Build history of the part. All positions in model axes, mm. Face numbers are marked on the shaded views. Round coordinates to 2 decimals unless told otherwise and drop trailing zeros. Order: outer loops, then holes, each group sorted by start corner. A loop starts at its lowest first (then second) coordinate and runs counter-clockwise, first axis right, second up. Notation, with made-up numbers: (77.5, 42.25) -> (81.5, 42.25) arc R10 cw to (81.5, 61.25) -> close; hole circle Ø8 at (69, 42.5). An arc over 180 degrees is marked (long way). Use a Markdown table: item, result. Add a question column.
Item 1: Two-plate mould, pull along Z, no slides. Class the marked faces 1, 2 and 3: released by +Z, released by -Z, zero draft, split by the parting line, or undercut.
Item 2: Slice it at A-A, the plane y = 0. Give the cut face in (x, z), plus the area to 3 significant figures.
Item 3: Slice it at D-D, the plane y = -13.5. Give the cut face in (x, z).
Item 4: Probe L1, parallel to Y at x = 32.5, z = 0; L2, parallel to X at y = -7, z = 15.5; L3, parallel to Y at x = 8, z = 2.5. List the from-to ranges inside material, lowest first.
Item 5: Pin check, flat tips, straight feed: pin 1 (1 mm diameter, centred on y = 2.5, z = -1.5, fed in from -X); pin 2 (4 mm diameter, centred on y = 1.5, z = 16, fed in from -X); pin 3 (6 mm diameter, centred on x = 23.5, z = -3, fed in from +Y); pin 4 (4 mm diameter, centred on x = 31.5, z = -4, fed in from -Y). Stop position of each tip, or through.
Item 6: Slice it at C-C, the plane x = 35. Give the cut face in (y, z), plus the area to 3 significant figures.
from build123d import *

# Parameters (mm, degrees)
SKETCH1_R           = 20
BOSS_EXTRUDE1_DEPTH = 40
SKETCH2_R           = 20
SKETCH2_R_2         = 5.5
CUT_EXTRUDE1_DEPTH  = 38
SKETCH3_R           = 3.5
CUT_EXTRUDE2_DEPTH  = 40


with BuildPart() as part:
    # Sketch1 → Boss-Extrude1 (new body)
    with BuildSketch(Plane(origin=(0, 0, 0), x_dir=(0, 0, -1), z_dir=(1, 0, 0))):
        Circle(SKETCH1_R)
    extrude(amount=BOSS_EXTRUDE1_DEPTH)

    # Sketch2 → Cut-Extrude1 (cut)
    with BuildSketch(Plane.ZY):
        Circle(SKETCH2_R)
        Circle(SKETCH2_R_2, mode=Mode.SUBTRACT)
    extrude(amount=-CUT_EXTRUDE1_DEPTH, mode=Mode.SUBTRACT)

    # Sketch3 → Cut-Extrude2 (cut)
    with BuildSketch(Plane.ZY):
        Circle(SKETCH3_R)
    extrude(amount=-CUT_EXTRUDE2_DEPTH, mode=Mode.SUBTRACT)


solid = part.part
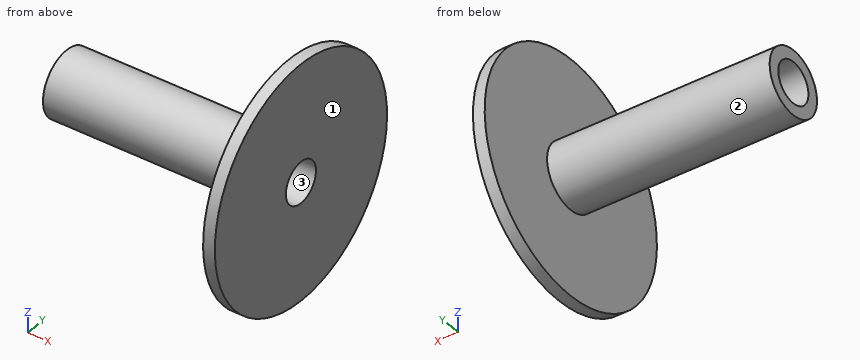
Check sheet entries:
| question | item | result |
|---|---|---|
| 1 | face 1 | zero draft |
| 1 | face 2 | split by the parting line |
| 1 | face 3 | undercut |
| 2 | outline | (0, -5.5) -> (38, -5.5) -> (38, -20) -> (40, -20) -> (40, -3.5) -> (0, -3.5) -> close; (0, 3.5) -> (40, 3.5) -> (40, 20) -> (38, 20) -> (38, 5.5) -> (0, 5.5) -> close |
| 2 | area | 218 mm2 |
| 3 | outline | (38, -14.76) -> (40, -14.76) -> (40, 14.76) -> (38, 14.76) -> close |
| 4 | L1 | -5.5 to -3.5, 3.5 to 5.5 |
| 4 | L2 | 38 to 40 |
| 4 | L3 | -4.9 to -2.45, 2.45 to 4.9 |
| 5 | pin 1 | through |
| 5 | pin 2 | x = 38 |
| 5 | pin 3 | y = 5.5 |
| 5 | pin 4 | y = -5.12 |
| 6 | outline | circle Ø11 at (0, 0); hole circle Ø7 at (0, 0) |
| 6 | area | 56.5 mm2 |
